Can you work these out from the drawing? Everything is in mm from the part's minimum corner. A direction names the side the tool comes from. Coordinates: 2 decimals unless noted, no trailing zeros. Loops run counter-clockwise (first coordinate to the right, second up) from the corner with the lowest first, then second, coordinate; pieces in that order, holes last.
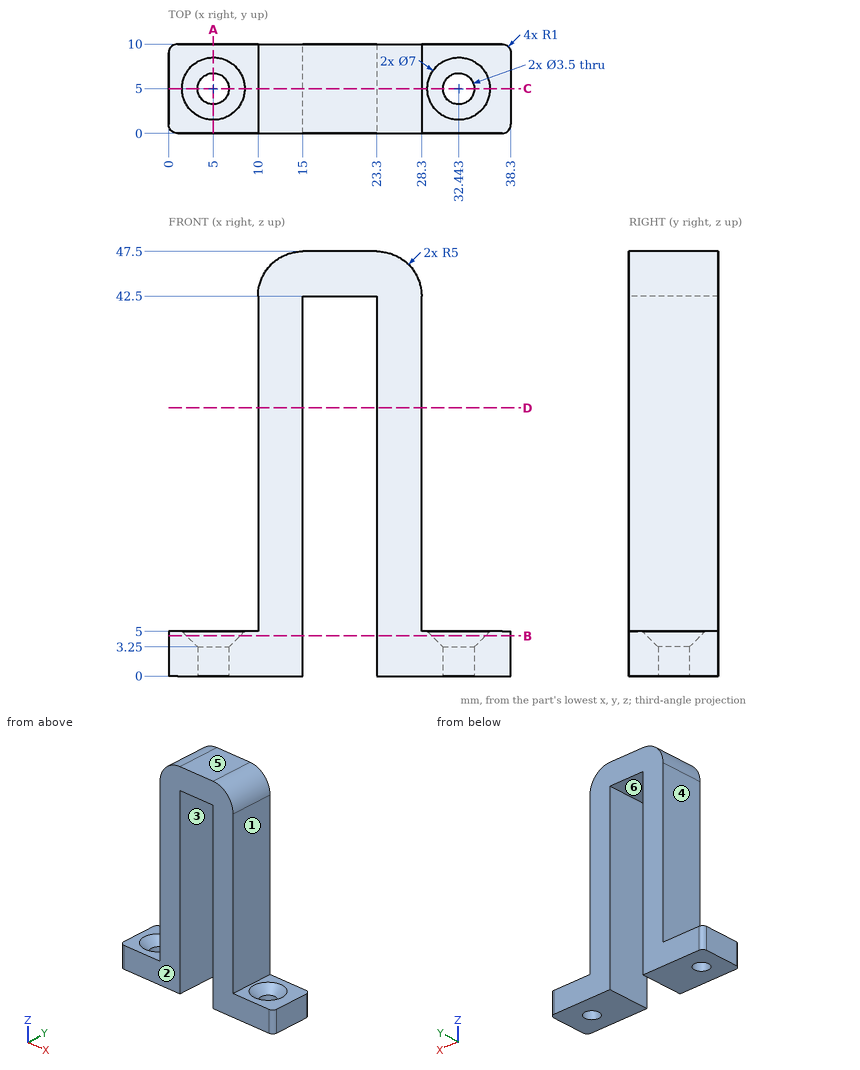
(1) Which directions (+Z, -Z, +X, -X, +Y, -Y) give clear straight access to the entire face, cutting with the end or side of a thin tool? Please do the marked faces 1, 2 and 3.
Answers:
face 1: +Z, +X, +Y, -Y
face 2: +Z, -Z, +X, -X, -Y
face 3: -Z, +Y, -Y
(2) Imagine slicing it at D-D, the plane z = 30. Write out the boundary of the cut face in (x, y).
Answers:
outline: (10, 0) - (15, 0) - (15, 10) - (10, 10) - close; (23.3, 0) - (28.3, 0) - (28.3, 10) - (23.3, 10) - close
(3) Imagine slicing it at B-B, the plane z = 4.5. Write out the boundary of the cut face in (x, y).
Answers:
outline: (0, 1) arc R1 ccw to (1, 0) - (15, 0) - (15, 10) - (1, 10) arc R1 ccw to (0, 9) - close; (23.3, 0) - (37.3, 0) arc R1 ccw to (38.3, 1) - (38.3, 9) arc R1 ccw to (37.3, 10) - (23.3, 10) - close; hole circle Ø6 at (5, 5); hole circle Ø6 at (32.44, 5)
(4) For pin 1 (4 mm diameter, centred on x = 18, y = 5, fed in from -Z); pin 2 (1.5 mm diameter, centred on x = 13, y = 1.5, fed in from +Z); pin 3 (5 mm diameter, centred on y = 5, z = 15.5, fed in from -X), each with a flat end and sliding along its axis, tell me the tip position at first contact or that it passes through.
Answers:
pin 1: stops at z = 42.5
pin 2: stops at z = 47.34
pin 3: stops at x = 10
(5) We'd pull the mould along X, two halves only. Please class the marked faces 4, 5 and 6: +X half, -X half, draft (parallel to the pull), parting line (faces both ways), or undercut.
Answers:
face 4: -X half
face 5: draft
face 6: undercut
(6) Imagine slicing it at C-C, the plane y = 5. Write out the boundary of the cut face in (x, z).
Answers:
outline: (0, 0) - (3.25, 0) - (3.25, 3.25) - (1.5, 5) - (0, 5) - close; (6.75, 0) - (15, 0) - (15, 42.5) - (23.3, 42.5) - (23.3, 0) - (30.69, 0) - (30.69, 3.25) - (28.94, 5) - (28.3, 5) - (28.3, 42.5) arc R5 ccw to (23.3, 47.5) - (15, 47.5) arc R5 ccw to (10, 42.5) - (10, 5) - (8.5, 5) - (6.75, 3.25) - close; (34.19, 0) - (38.3, 0) - (38.3, 5) - (35.94, 5) - (34.19, 3.25) - close
(7) I need wall thicknesses on probe 1 along X at (y, z) = (5, 1.65); probe 2 along X at (y, z) = (4, 31); probe 3 along Y at (x, z) = (5, 1). Which ranges of each line are inside material? Lowest first, please.
Answers:
probe 1: x = 0 to 3.25, 6.75 to 15, 23.3 to 30.69, 34.19 to 38.3
probe 2: x = 10 to 15, 23.3 to 28.3
probe 3: y = 0 to 3.25, 6.75 to 10
(8) Imagine slicing it at A-A, the plane x = 5. Write out the boundary of the cut face in (y, z).
Answers:
outline: (0, 0) - (3.25, 0) - (3.25, 3.25) - (1.5, 5) - (0, 5) - close; (6.75, 0) - (10, 0) - (10, 5) - (8.5, 5) - (6.75, 3.25) - close
